```python
from build123d import *

# Parameters (mm, degrees)
F1_DEPTH    = 19.05
F2_T1_DEPTH = 165.1
F2_T3_DEPTH = 165.1


# Not quite as in the source:
# - a fillet or chamfer that OpenCascade refuses, or shapes differently, is made with other operations: its cross-section is extruded or revolved along the edge and cut away or added
# - a feature names something its author has since deleted; it is built from what else it names


with BuildPart() as f1:
    # F0 (on Right) → F1 (new body)
    with BuildSketch(Plane.YZ):
        Polygon((-36.6194384832, 94.9639305791), (3.7774763688, 1.7402786959), (44.5628240677, 19.4139289437), (4.1659092157, 112.6375808269), align=None)
    extrude(amount=F1_DEPTH)

    # F2: fillet of radius 12.7 on 4 edges, made by hand

    # F2_s2 → F2_t1 (cut)
    with BuildSketch(Plane(origin=(0, 12.5863228888, -29.0453612057), x_dir=(1, 0, 0), z_dir=(0, -0.3976074296, 0.9175556288))):
        with BuildLine():
            ThreePointArc((12.7, 48.6079924439), (3.7197438789, 44.888248565), (0, 35.9079924439))
            Line((0, 35.9079924439), (0, 48.6079924439))
            Line((0, 48.6079924439), (12.7, 48.6079924439))
        make_face()
        with BuildLine():
            ThreePointArc((6.35, 48.6079924439), (15.3302561211, 44.888248565), (19.05, 35.9079924439))
            Line((19.05, 35.9079924439), (19.05, 48.6079924439))
            Line((19.05, 48.6079924439), (6.35, 48.6079924439))
        make_face()
    extrude(amount=F2_T1_DEPTH, mode=Mode.SUBTRACT)

    # F2_s4 → F2_t3 (cut)
    with BuildSketch(Plane(origin=(0, -53.0586637457, 122.4430731045), x_dir=(1, 0, 0), z_dir=(0, 0.3976074296, -0.9175556288))):
        with BuildLine():
            ThreePointArc((12.7, -4.1579924439), (3.7197438789, -7.8777363228), (0, -16.8579924439))
            Line((0, -16.8579924439), (0, -4.1579924439))
            Line((0, -4.1579924439), (12.7, -4.1579924439))
        make_face()
        with BuildLine():
            ThreePointArc((6.35, -4.1579924439), (15.3302561211, -7.8777363228), (19.05, -16.8579924439))
            Line((19.05, -16.8579924439), (19.05, -4.1579924439))
            Line((19.05, -4.1579924439), (6.35, -4.1579924439))
        make_face()
    extrude(amount=F2_T3_DEPTH, mode=Mode.SUBTRACT)


solid = f1.part
```
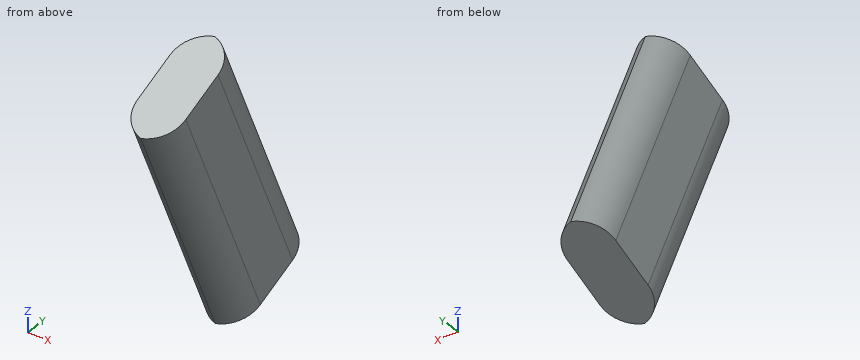
Design review of the part built by this model. Coordinates are the model's own, in mm. Give positions to 0.01 mm unless a question says otherwise; leave off trailing zeros. Order: outer loops, then holes, each group sorted by start corner. A loop starts at its lowest first (then second) coordinate and runs counter-clockwise, first axis right, second up. Notation, with made-up numbers: (10.25, 0.25) - (29.25, 0.25) arc R10 ccw to (29.25, 6.25) - close; hole circle Ø7 at (69.5, -40). An arc over 180 degrees is marked (long way). Use a Markdown table: item, result. Add a question column.
(1) Add section B-B on x = 15.25. Give the boundary of the cut face in (y, z).
(2) Wall thickness on probe 1 along Y at (x, z) = (13.25, 73.5); probe 2 along Z at (x, y) = (13.5, 12.5); probe 3 along Y at (x, z) = (12.5, 53.5): over which ranges is each line inside the solid? List them lowest first. Write a range as [from, to].
(3) Add section A-A on x = 4.5. Give the boundary of the cut face in (y, z), then the cut area to 3 significant figures.
(4) Clearance check with flat-ended pins moving along their axes: P1, Ø1.5, axis at x = 10.5, z = 41, coming from the +Y side; P2, Ø2, axis at y = -0.5, z = 20.5, coming from the -X side; P3, Ø6, axis at x = 3, z = 40, coming from the -Y side; P4, Ø12, axis at y = -22.5, z = 34, coming from the -X side. State where each tip first meets the part, or that it passes through.
Report:
| question | item | result |
|---|---|---|
| 1 | outline | (-33.28, 96.41) - (7.12, 3.19) - (41.22, 17.97) - (0.83, 111.19) - close |
| 2 | probe 1 | y = [-25.1, 18.9] |
| 2 | probe 2 | z = [5.52, 87.86] |
| 2 | probe 3 | y = [-16.92, 28.06] |
| 3 | outline | (-33.86, 96.16) - (6.53, 2.93) - (41.81, 18.22) - (1.41, 111.44) - close |
| 3 | area | 3,910 mm² |
| 4 | P1 | stops at y = 34.87 |
| 4 | P2 | stops at x = 2.97 |
| 4 | P3 | stops at y = -11.09 |
| 4 | P4 | passes through |
